```python
from build123d import *

# Parameters (mm, degrees)
SKETCH_W               = 358.3
SKETCH_H               = 64
PAD_DEPTH              = 15
SKETCH001_W            = 358.3
SKETCH001_H            = 4
POCKET_DEPTH           = 7.5
SKETCH002_R            = 1.5
POCKET001_DEPTH        = 20
SKETCH003_R            = 1.5
POCKET002_DEPTH        = 20
POCKET003_DEPTH        = 7.5
POCKET004_DEPTH        = 3.75
LINEARPATTERN_COUNT    = 5
LINEARPATTERN_PITCH    = 70.2
POCKET005_DEPTH        = 739.810922
LINEARPATTERN001_COUNT = 5
LINEARPATTERN001_PITCH = 70.2


with BuildPart() as part:
    # Sketch → Pad (new body)
    with BuildSketch(Plane.YZ):
        with Locations((179.15, 32)):
            Rectangle(SKETCH_W, SKETCH_H)
    extrude(amount=PAD_DEPTH)

    # Sketch001 (on Face5 of Pad) → Pocket (cut)
    with BuildSketch(Plane(origin=(0, 0, 0), x_dir=(0, 1, 0), z_dir=(-1, 0, 0))):
        with Locations((179.15, -22)):
            Rectangle(SKETCH001_W, SKETCH001_H)
    extrude(amount=-POCKET_DEPTH, mode=Mode.SUBTRACT)

    # Sketch002 (on Face3 of Pocket) → Pocket001 (cut)
    with BuildSketch(Plane(origin=(0, 0, 0), x_dir=(0, 0, -1), z_dir=(0, -1, 0))):
        with Locations((-56.5, 7.5)):
            Circle(SKETCH002_R)
        with Locations((-31.5, 7.5)):
            Circle(SKETCH002_R)
        with Locations((-10, 7.5)):
            Circle(SKETCH002_R)
    extrude(amount=-POCKET001_DEPTH, mode=Mode.SUBTRACT)

    # Sketch003 (on Face2 of Pocket001) → Pocket002 (cut)
    with BuildSketch(Plane.ZX.offset(358.3)):
        with Locations((10, 7.5)):
            Circle(SKETCH003_R)
        with Locations((31.5, 7.5)):
            Circle(SKETCH003_R)
        with Locations((56.5, 7.5)):
            Circle(SKETCH003_R)
    extrude(amount=-POCKET002_DEPTH, mode=Mode.SUBTRACT)

    # Sketch004 (on Face5 of Pocket002) → Pocket003 (cut)
    with BuildSketch(Plane.YZ.offset(15)):
        Polygon((0, 36.5), (358.3, 36.5), (358.3, 51.5), (0, 51.5), (0, 44), align=None)
    extrude(amount=-POCKET003_DEPTH, mode=Mode.SUBTRACT)

    # Sketch005 (on Face5 of Pocket003) → Pocket004 (cut)
    with BuildSketch(Plane.YZ.offset(15)):
        with BuildLine():
            Line((46.3, 34.5), (46.3, 0))
            Line((46.3, 0), (31.3, 0))
            Line((31.3, 0), (31.3, 34.5))
            ThreePointArc((31.3, 34.5), (30.714214, 35.914214), (29.3, 36.5))
            Line((29.3, 36.5), (48.3, 36.5))
            ThreePointArc((48.3, 36.5), (46.885786, 35.914214), (46.3, 34.5))
        make_face()
    pocket004 = extrude(amount=-POCKET004_DEPTH, mode=Mode.SUBTRACT)

    # LinearPattern: Pocket004 ×5
    with Locations(*[(0, i * LINEARPATTERN_PITCH, 0) for i in range(1, LINEARPATTERN_COUNT)]):
        add(pocket004, mode=Mode.SUBTRACT)

    # Sketch006 (on Face6 of MultiTransform) → Pocket005 (cut, through all)
    with BuildSketch(Plane.YZ.offset(11.25)):
        with BuildLine():
            Line((31.3, 0), (46.3, 0))
            Line((46.3, 0), (46.3, 4.666667))
            ThreePointArc((46.3, 4.666667), (45.714214, 6.08088), (44.3, 6.666667))
            Line((44.3, 6.666667), (33.3, 6.666667))
            ThreePointArc((33.3, 6.666667), (31.885786, 6.08088), (31.3, 4.666667))
            Line((31.3, 4.666667), (31.3, 0))
        make_face()
    pocket005 = extrude(amount=-POCKET005_DEPTH, mode=Mode.SUBTRACT)

    # LinearPattern001: Pocket005 ×5
    with Locations(*[(0, i * LINEARPATTERN001_PITCH, 0) for i in range(1, LINEARPATTERN001_COUNT)]):
        add(pocket005, mode=Mode.SUBTRACT)


solid = part.part
```
Build history of the part. All positions in model axes, mm. A direction names the side the tool comes from. Round coordinates to 2 decimals unless told otherwise and drop trailing zeros. Order: outer loops, then holes, each group sorted by start corner. A loop starts at its lowest first (then second) coordinate and runs counter-clockwise, first axis right, second up. Notation, with made-up numbers: (-19, -28) -> (9, -28) arc R12 ccw to (9, -23) -> close; hole circle Ø7 at (-10, 85.5). An arc over 180 degrees is marked (long way). Answer in a Markdown table with one row per item.
1) Pin check, flat tips, straight feed: P1, Ø9.5, axis at y = 177, z = 28, coming from the +X side; P2, Ø0.9, axis at x = 7, z = 31.5, coming from the +Y side; P3, Ø1.2, axis at y = 227, z = 21.5, coming from the -X side. Stop position of each tip, or through.
Values:
| item | result |
|---|---|
| P1 | x = 11.25 |
| P2 | y = 338.3 |
| P3 | x = 7.5 |
2) Band-saw the part on A-A on z = 16. Give the cut face in (x, y).
Values:
| item | result |
|---|---|
| outline | (0, 0) -> (15, 0) -> (15, 31.3) -> (11.25, 31.3) -> (11.25, 46.3) -> (15, 46.3) -> (15, 101.5) -> (11.25, 101.5) -> (11.25, 116.5) -> (15, 116.5) -> (15, 171.7) -> (11.25, 171.7) -> (11.25, 186.7) -> (15, 186.7) -> (15, 241.9) -> (11.25, 241.9) -> (11.25, 256.9) -> (15, 256.9) -> (15, 312.1) -> (11.25, 312.1) -> (11.25, 327.1) -> (15, 327.1) -> (15, 358.3) -> (0, 358.3) -> close |
3) Band-saw the part on C-C on z = 44.5. Give the cut face in (x, y), and give its area (3 significant figures).
Values:
| item | result |
|---|---|
| outline | (0, 0) -> (7.5, 0) -> (7.5, 358.3) -> (0, 358.3) -> close |
| area | 2,690 mm2 |
4) Mould opens along Z. For faces 1 (the flat face through (12, 101.5, 12)), 2 (the flat face through (4, 177, 20)), 3 (the flat face through (7, 74, 0)) say: released by +Z, released by -Z, zero draft, split by the parting line, or undercut.
Values:
| item | result |
|---|---|
| face 1 | zero draft |
| face 2 | undercut |
| face 3 | released by -Z |
5) Which spindle directions (+Z, -Z, +X, -X, +Y, -Y) get a long thin tool onto all of the face, cutting with end or side? Do faces 4 (the flat face through (12, 241.9, 12)), 5 (the flat face through (6, 109, 6.667)), 6 (the flat face through (10, 177, 36.5)). Say none if no direction does.
Values:
| item | result |
|---|---|
| face 4 | -Z, +X |
| face 5 | -Z, +X, -X |
| face 6 | +X, +Y, -Y |
6) Band-saw the part on B-B on y = 297. Give the cut face in (x, z), and give its area (4 significant figures).
Values:
| item | result |
|---|---|
| outline | (0, 0) -> (15, 0) -> (15, 36.5) -> (7.5, 36.5) -> (7.5, 51.5) -> (15, 51.5) -> (15, 64) -> (0, 64) -> (0, 24) -> (7.5, 24) -> (7.5, 20) -> (0, 20) -> close |
| area | 817.5 mm2 |
7) Wall check: L1, parallel to Y at x = 12.5, z = 6; L2, parallel to Z at x = 11.5, y = 138.5; L3, parallel to X at y = 7, z = 10. Give the ranges that are in metal, low to high.
Values:
| item | result |
|---|---|
| L1 | 0 to 31.3, 46.3 to 101.5, 116.5 to 171.7, 186.7 to 241.9, 256.9 to 312.1, 327.1 to 358.3 |
| L2 | 0 to 36.5, 51.5 to 64 |
| L3 | 0 to 6, 9 to 15 |
